The listing builds one solid part. Answer for the finished solid, in the listing's coordinates (mm). Face numbers are marked on the shaded views. A direction names the side the tool comes from. Round coordinates to 2 decimals unless told otherwise and drop trailing zeros. Loops run counter-clockwise (first coordinate to the right, second up) from the corner with the lowest first, then second, coordinate; pieces in that order, holes last. Notation, with made-up numbers: M 12.25,21.5 L 39.25,21.5 A30 ccw 39.25,49.5 Z; hole C 64,62.5 d8. An arc over 180 degrees is marked long. Answer as a JSON object with one key per item and string values.
```python
from build123d import *

# Parameters (mm, degrees)
SKETCH_1_R      = 25
SKETCH_1_R_2    = 2.1
EXTRUDE_1_DEPTH = 5
SKETCH_2_R      = 25
SKETCH_2_R_2    = 24
SKETCH_2_R_3    = 12
EXTRUDE_2_DEPTH = 4
FILLET_1_R      = 1
SKETCH_3_R      = 8
EXTRUDE_3_DEPTH = 30
SKETCH_4_R      = 2.1
EXTRUDE_5_DEPTH = 6


with BuildPart() as part:
    # Эскиз1 → Бобышка-Вытянуть1 (new body)
    with BuildSketch(Plane(origin=(0, 0, 0), x_dir=(1, 0, 0), z_dir=(0, 1, 0))):
        with Locations(Location((0, 0, 0), (0, 0, 270))):
            Circle(SKETCH_1_R)
        with Locations(Location((-18, 0, 0), (0, 0, 270))):
            Circle(SKETCH_1_R_2, mode=Mode.SUBTRACT)
        with Locations(Location((-12.727922061, 12.727922061, 0), (0, 0, 270))):
            Circle(SKETCH_1_R_2, mode=Mode.SUBTRACT)
        with Locations(Location((0, 18, 0), (0, 0, 270))):
            Circle(SKETCH_1_R_2, mode=Mode.SUBTRACT)
        with Locations(Location((12.727922061, 12.727922061, 0), (0, 0, 270))):
            Circle(SKETCH_1_R_2, mode=Mode.SUBTRACT)
        with Locations(Location((18, 0, 0), (0, 0, 270))):
            Circle(SKETCH_1_R_2, mode=Mode.SUBTRACT)
        with Locations(Location((12.727922061, -12.727922061, 0), (0, 0, 270))):
            Circle(SKETCH_1_R_2, mode=Mode.SUBTRACT)
        with Locations(Location((0, -18, 0), (0, 0, 270))):
            Circle(SKETCH_1_R_2, mode=Mode.SUBTRACT)
        with Locations(Location((-12.727922061, -12.727922061, 0), (0, 0, 270))):
            Circle(SKETCH_1_R_2, mode=Mode.SUBTRACT)
    extrude(amount=EXTRUDE_1_DEPTH)

    # Эскиз2 → Бобышка-Вытянуть2 (add)
    # profile 1 of 10: a face of its own
    with BuildSketch(Plane(origin=(0, 5, 0), x_dir=(1, 0, 0), z_dir=(0, 1, 0))):
        with Locations(Location((0, 0, 0), (0, 0, 270))):
            Circle(SKETCH_2_R)
        Circle(SKETCH_2_R_2, mode=Mode.SUBTRACT)
    # profile 2 of 10: a face of its own
    with BuildSketch(Plane(origin=(0, 5, 0), x_dir=(1, 0, 0), z_dir=(0, 1, 0))):
        Circle(SKETCH_2_R_3)
    # profile 3 of 10: a face of its own
    with BuildSketch(Plane(origin=(0, 5, 0), x_dir=(1, 0, 0), z_dir=(0, 1, 0))):
        with BuildLine():
            Line((-10.332266323, 21.662046824), (-5.166133162, 10.831023412))
            ThreePointArc((-5.166133162, 10.831023412), (-4.592201188, 11.08655439), (-4.005682311, 11.311697893))
            Line((-4.005682311, 11.311697893), (-8.011364622, 22.623395786))
            ThreePointArc((-8.011364622, 22.623395786), (-9.184402377, 22.17310878), (-10.332266323, 21.662046824))
        make_face()
    # profile 4 of 10: a face of its own
    with BuildSketch(Plane(origin=(0, 5, 0), x_dir=(1, 0, 0), z_dir=(0, 1, 0))):
        with BuildLine():
            Line((8.011364622, 22.623395786), (4.005682311, 11.311697893))
            ThreePointArc((4.005682311, 11.311697893), (4.592201188, 11.08655439), (5.166133162, 10.831023412))
            Line((5.166133162, 10.831023412), (10.332266323, 21.662046824))
            ThreePointArc((10.332266323, 21.662046824), (9.184402377, 22.17310878), (8.011364622, 22.623395786))
        make_face()
    # profile 5 of 10: a face of its own
    with BuildSketch(Plane(origin=(0, 5, 0), x_dir=(1, 0, 0), z_dir=(0, 1, 0))):
        with BuildLine():
            ThreePointArc((10.831023412, 5.166133162), (11.08655439, 4.592201188), (11.311697893, 4.005682311))
            Line((11.311697893, 4.005682311), (22.623395786, 8.011364622))
            ThreePointArc((22.623395786, 8.011364622), (22.17310878, 9.184402377), (21.662046824, 10.332266323))
            Line((21.662046824, 10.332266323), (10.831023412, 5.166133162))
        make_face()
    # profile 6 of 10: a face of its own
    with BuildSketch(Plane(origin=(0, 5, 0), x_dir=(1, 0, 0), z_dir=(0, 1, 0))):
        with BuildLine():
            ThreePointArc((11.311697893, -4.005682311), (11.08655439, -4.592201188), (10.831023412, -5.166133162))
            Line((10.831023412, -5.166133162), (21.662046824, -10.332266323))
            ThreePointArc((21.662046824, -10.332266323), (22.17310878, -9.184402377), (22.623395786, -8.011364622))
            Line((22.623395786, -8.011364622), (11.311697893, -4.005682311))
        make_face()
    # profile 7 of 10: a face of its own
    with BuildSketch(Plane(origin=(0, 5, 0), x_dir=(1, 0, 0), z_dir=(0, 1, 0))):
        with BuildLine():
            ThreePointArc((5.166133162, -10.831023412), (4.592201188, -11.08655439), (4.005682311, -11.311697893))
            Line((4.005682311, -11.311697893), (8.011364622, -22.623395786))
            ThreePointArc((8.011364622, -22.623395786), (9.184402377, -22.17310878), (10.332266323, -21.662046824))
            Line((10.332266323, -21.662046824), (5.166133162, -10.831023412))
        make_face()
    # profile 8 of 10: a face of its own
    with BuildSketch(Plane(origin=(0, 5, 0), x_dir=(1, 0, 0), z_dir=(0, 1, 0))):
        with BuildLine():
            ThreePointArc((-4.005682311, -11.311697893), (-4.592201188, -11.08655439), (-5.166133162, -10.831023412))
            Line((-5.166133162, -10.831023412), (-10.332266323, -21.662046824))
            ThreePointArc((-10.332266323, -21.662046824), (-9.184402377, -22.17310878), (-8.011364622, -22.623395786))
            Line((-8.011364622, -22.623395786), (-4.005682311, -11.311697893))
        make_face()
    # profile 9 of 10: a face of its own
    with BuildSketch(Plane(origin=(0, 5, 0), x_dir=(1, 0, 0), z_dir=(0, 1, 0))):
        with BuildLine():
            Line((-21.662046824, -10.332266323), (-10.831023412, -5.166133162))
            ThreePointArc((-10.831023412, -5.166133162), (-11.08655439, -4.592201188), (-11.311697893, -4.005682311))
            Line((-11.311697893, -4.005682311), (-22.623395786, -8.011364622))
            ThreePointArc((-22.623395786, -8.011364622), (-22.17310878, -9.184402377), (-21.662046824, -10.332266323))
        make_face()
    # profile 10 of 10: a face of its own
    with BuildSketch(Plane(origin=(0, 5, 0), x_dir=(1, 0, 0), z_dir=(0, 1, 0))):
        with BuildLine():
            Line((-22.623395786, 8.011364622), (-11.311697893, 4.005682311))
            ThreePointArc((-11.311697893, 4.005682311), (-11.08655439, 4.592201188), (-10.831023412, 5.166133162))
            Line((-10.831023412, 5.166133162), (-21.662046824, 10.332266323))
            ThreePointArc((-21.662046824, 10.332266323), (-22.17310878, 9.184402377), (-22.623395786, 8.011364622))
        make_face()
    extrude(amount=EXTRUDE_2_DEPTH)

    # Скругление1
    fillet_1_edges = [part.edges().sort_by_distance(p)[0] for p in [
        (5.166133162, 7, 10.831023412),
        (10.831023412, 7, 5.166133162),
        (21.662046824, 7, 10.332266323),
        (22.623395786, 7, 8.011364622),
        (11.311697893, 7, 4.005682311),
        (11.311697893, 7, -4.005682311),
        (21.662046824, 7, -10.332266323),
        (10.831023412, 7, -5.166133162),
        (5.166133162, 7, -10.831023412),
        (8.011364622, 7, -22.623395786),
        (4.005682311, 7, -11.311697893),
        (-4.005682311, 7, -11.311697893),
        (-10.332266323, 7, -21.662046824),
        (-5.166133162, 7, -10.831023412),
        (-10.831023412, 7, -5.166133162),
        (-22.623395786, 7, -8.011364622),
        (-11.311697893, 7, -4.005682311),
        (-11.311697893, 7, 4.005682311),
        (-21.662046824, 7, 10.332266323),
        (-10.831023412, 7, 5.166133162),
        (-5.166133162, 7, 10.831023412),
        (-8.011364622, 7, 22.623395786),
        (-4.005682311, 7, 11.311697893),
        (4.005682311, 7, 11.311697893),
        (10.332266323, 7, 21.662046824),
        (22.623395786, 7, -8.011364622),
        (10.332266323, 7, -21.662046824),
        (-8.011364622, 7, -22.623395786),
        (-21.662046824, 7, -10.332266323),
        (-22.623395786, 7, 8.011364622),
        (-10.332266323, 7, 21.662046824),
        (8.011364622, 7, 22.623395786),
    ]]
    fillet(fillet_1_edges, radius=FILLET_1_R)

    # Эскиз3 → Бобышка-Вытянуть3 (add)
    with BuildSketch(Plane(origin=(0, 9, 0), x_dir=(1, 0, 0), z_dir=(0, 1, 0))):
        with Locations(Location((0, 0, 0), (0, 0, 270))):
            Circle(SKETCH_3_R)
    extrude(amount=EXTRUDE_3_DEPTH)

    # Эскиз4 → Бобышка-Вытянуть5 (add)
    with BuildSketch(Plane(origin=(0, 39, 0), x_dir=(1, 0, 0), z_dir=(0, 1, 0))):
        Polygon((5, -20), (5, -5), (20, -5), (20, 5.110143601), (5, 5.110143601), (5, 20), (-5, 20), (-5, 5.280605092), (-20, 5.280605092), (-20, -5), (-5, -5), (-5, -20), align=None)
        with Locations(Location((15, 0, 0), (0, 0, 270))):
            Circle(SKETCH_4_R, mode=Mode.SUBTRACT)
        with Locations(Location((0, 15, 0), (0, 0, 270))):
            Circle(SKETCH_4_R, mode=Mode.SUBTRACT)
        with Locations(Location((-15, 0, 0), (0, 0, 270))):
            Circle(SKETCH_4_R, mode=Mode.SUBTRACT)
        with Locations(Location((0, -15, 0), (0, 0, 270))):
            Circle(SKETCH_4_R, mode=Mode.SUBTRACT)
    extrude(amount=-EXTRUDE_5_DEPTH)


solid = part.part
```
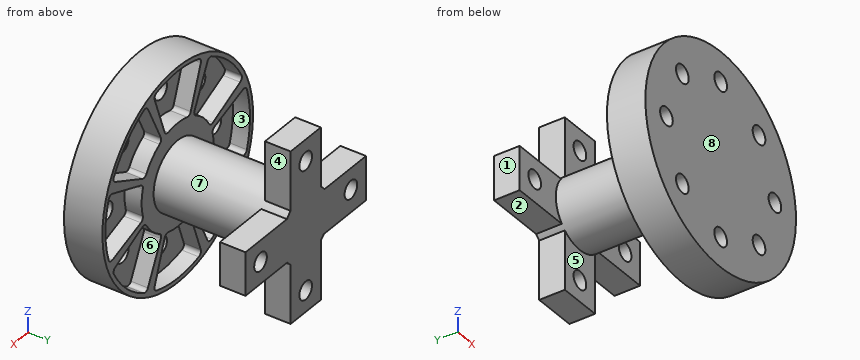
Item 1: The part is cut by section B-B (z = 9). Give the vertices of the cut face in (x, y), then the cut area to 3 significant figures.
Values follow:
{"outline": "M -23.32,0 L 23.32,0 L 23.32,9 L 18.87,9 L 18.87,5 L 7.94,5 L 7.94,9 L -7.94,9 L -7.94,5 L -18.87,5 L -18.87,9 L -23.32,9 Z; M -5,33 L 5,33 L 5,39 L -5,39 Z", "area": "392 mm^2"}
Item 2: Flat-ended cylindrical pins translate along their axes: P1, Ø12.5, axis at x = -11.5, z = 13, coming from the +Y side; P2, Ø8, axis at y = 5.5, z = -17, coming from the +X side; P3, Ø3, axis at x = 0, y = 35, coming from the -Z side. Find the tip coordinate at first contact, or state that the pin passes through.
Values follow:
{"P1": "y = 9", "P2": "x = 21.35", "P3": "z = -20"}
Item 3: Determine the mould class of the marked faces 5, 6, 7 and 8 for opening direction Y: released by +Y, released by -Y, zero draft, split by the parting line, or undercut.
Values follow:
{"face 5": "undercut", "face 6": "zero draft", "face 7": "undercut", "face 8": "released by -Y"}
Item 4: Which of the six approach directions +Z, -Z, +X, -X, +Y, -Y give full straight-line access (tool end or side, diameter ignored) to the marked faces 1, 2, 3 and 4?
Values follow:
{"face 1": "+Z, -Z, -X, +Y", "face 2": "-Z, -X, +Y", "face 3": "+Y", "face 4": "+Z, +X, +Y"}
Item 5: The part is cut by section A-A (x = 18). Give the vertices of the cut face in (y, z), then the cut area to 3 significant figures.
Values follow:
{"outline": "M 0,-17.35 L 9,-17.35 L 9,-15.87 L 5,-15.87 L 5,-8.59 L 9,-8.59 L 9,-6.37 L 5,-6.37 L 5,-2.1 L 0,-2.1 Z; M 0,2.1 L 5,2.1 L 5,6.37 L 9,6.37 L 9,8.59 L 5,8.59 L 5,15.87 L 9,15.87 L 9,17.35 L 0,17.35 Z; M 33,-5.11 L 39,-5.11 L 39,5 L 33,5 Z", "area": "243 mm^2"}
Item 6: The part is cut by section D-D (x = 0). Give the number of separate pieces and of enclosed holes in the cut face, then the cut area to 3 significant figures.
Values follow:
{"separate pieces": "5", "enclosed holes": "0", "area": "886 mm^2"}
Item 7: The part is cut by section C-C (z = 18). Give the vertices of the cut face in (x, y), then the cut area to 3 significant figures.
Values follow:
{"outline": "M -17.35,0 L -2.1,0 L -2.1,5 L -6.37,5 L -6.37,9 L -8.59,9 L -8.59,5 L -15.87,5 L -15.87,9 L -17.35,9 Z; M -5,33 L 5,33 L 5,39 L -5,39 Z; M 2.1,0 L 17.35,0 L 17.35,9 L 15.87,9 L 15.87,5 L 8.59,5 L 8.59,9 L 6.37,9 L 6.37,5 L 2.1,5 Z", "area": "242 mm^2"}
Item 8: Straight lines are drawn through the part: line 1 (X direction, y = 3.9, z = 0); line 2 (X direction, y = 37, z = 0); line 3 (X direction, y = 35.45, z = -15). For each, find the intervals that lie inside material, in ascending order.
Values follow:
{"line 1": "-25 to -20.1, -15.9 to 15.9, 20.1 to 25", "line 2": "-20 to -17.1, -12.9 to 12.9, 17.1 to 20", "line 3": "-5 to -2.1, 2.1 to 5"}
